Here's the drawing with two shaded views (mm, measured from the low corner). I have some questions. Round coordinates to 2 decimals unless told otherwise and drop trailing zeros. Order: outer loops, then holes, each group sorted by start corner. A loop starts at its lowest first (then second) coordinate and runs counter-clockwise, first axis right, second up.
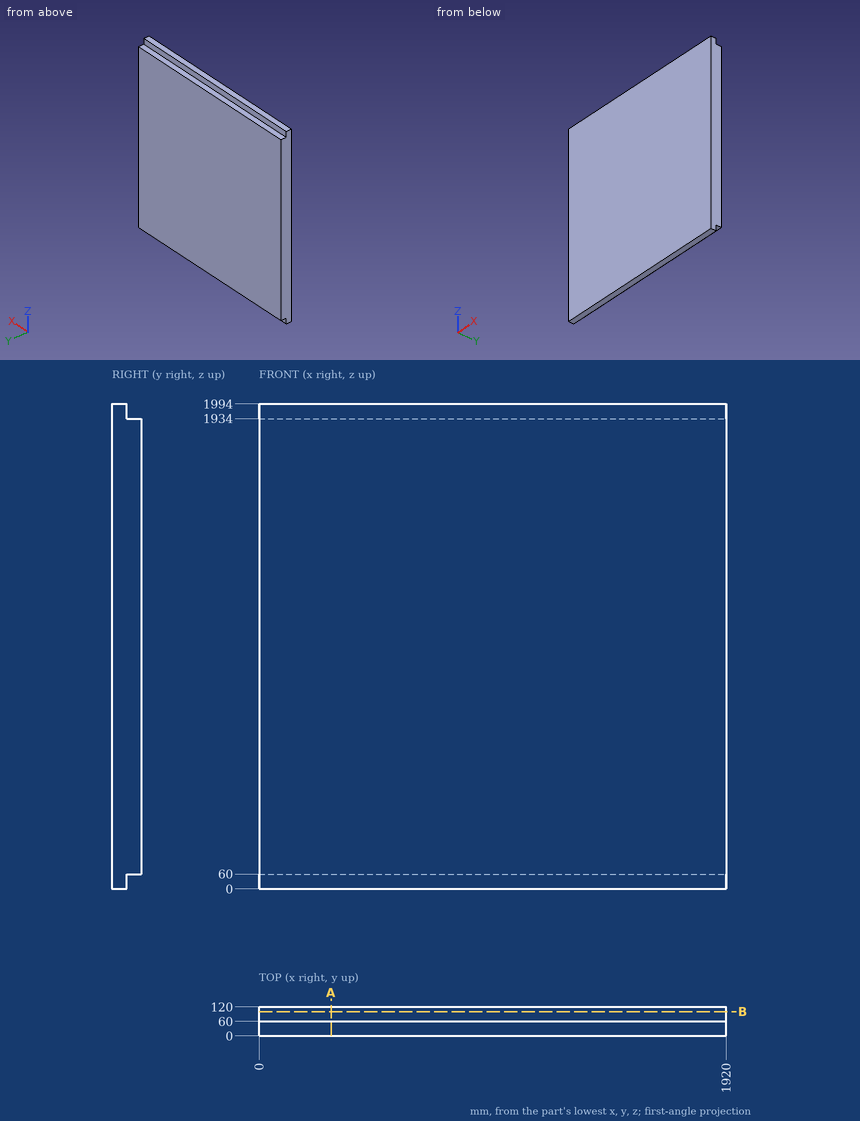
1. If we section it at B-B, the plane y = 100: Write out the boundary of the cut face in (x, z).
Evaluation:
outline: (0, 60) - (1920, 60) - (1920, 1934) - (0, 1934) - close
2. I'm going to push flat-ended pins straight in: P1, Ø18, axis at x = 819.5, z = 1954, coming from the +Y side; P2, Ø12, axis at x = 574.5, y = 107, coming from the +Z side; P3, Ø1.5, axis at x = 842.5, y = 102, coming from the -Z side. Where does each tip first touch, or does it pass through?
Evaluation:
P1: stops at y = 60
P2: stops at z = 1934
P3: stops at z = 60
3. If we section it at A-A, the plane x = 295.5: Write out the boundary of the cut face in (y, z).
Evaluation:
outline: (0, 0) - (60, 0) - (60, 60) - (120, 60) - (120, 1934) - (60, 1934) - (60, 1994) - (0, 1994) - close
4. I need wall thicknesses on probe 1 along Z at (x, y) = (970, 101). Which ranges of the line are inside material? Lowest first, please.
Evaluation:
probe 1: z = 60 to 1934
